CAD build for the part. Positions are in the model's coordinates, mm. Give positions to 0.01 mm unless a question says otherwise; leave off trailing zeros. Loops run counter-clockwise (first coordinate to the right, second up) from the corner with the lowest first, then second, coordinate; pieces in that order, holes last.
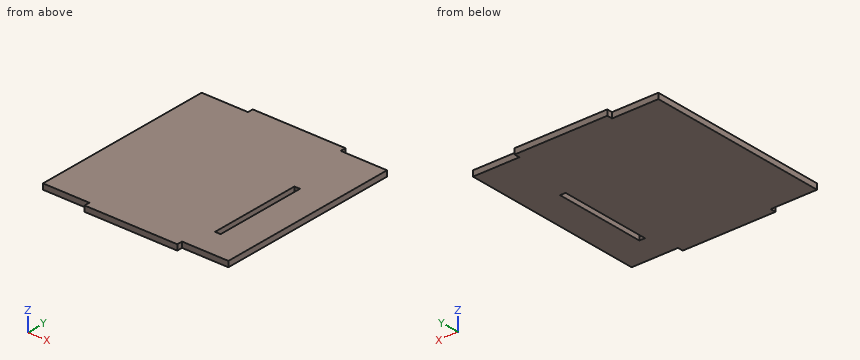
Autodesk Inventor part; units mm, degrees
ref_plane "YZ Plane" through (0, 0, 0) normal (1, 0, 0) x (0, 1, 0)
ref_plane "XZ Plane" through (0, 0, 0) normal (0, 1, 0) x (-1, 0, 0)
ref_plane "XY Plane" through (0, 0, 0) normal (0, 0, 1) x (1, 0, 0)
sketch "Boceto1" plane through (0, 0, 0) normal (0, 0, 1) x (1, 0, 0)
  line L0 (0, 100) -> (0, 0)
  line L1 (-75, 0) -> (-75, -3)
  line L2 (-75, -3) -> (-25, -3)
  line L3 (-25, -3) -> (-25, 0)
  line L4 (0, 0) -> (-25, 0)
  line L5 (-100, 0) -> (-75, 0)
  line L6 (-75, 100) -> (-75, 103)
  line L7 (-75, 103) -> (-25, 103)
  line L8 (-25, 103) -> (-25, 100)
  line L9 (0, 100) -> (-25, 100)
  line L10 (-75, 100) -> (-100, 100)
  line L11 (-100, 100) -> (-100, 0)
  dimension "d1" = 100
  dimension "d4" = 50
  dimension "d5" = 25
  dimension "d10" = 3
  dimension "d13" = 50
  dimension "d14" = 3
  dimension "d37" = 100
extrude "Extrusión2" add sketch "Boceto1" along normal blind 3
sketch "Boceto2" plane through (0, 0, 3) normal (0, 0, 1) x (1, 0, 0)
  line L0 (-20, 65) -> (-17, 65)
  line L1 (-17, 65) -> (-17, 15)
  line L2 (-17, 15) -> (-20, 15)
  line L3 (-20, 15) -> (-20, 65)
  line L4 (-25, 0) -> (0, 0)
  line L5 (-100, 100) -> (-100, 0)
  dimension "d38" = 3
  dimension "d39" = 50
  dimension "d40" = 15
  dimension "d41" = 80
extrude "Extrusión3" cut sketch "Boceto2" against normal blind 3
properties part number "Control lateral"
1. Drop flat-ended pins along their axis: pin 1 (0.9 mm diameter, centred on x = -17, z = 1.5, fed in from +Y); pin 2 (1.5 mm diameter, centred on y = 102, z = 1.5, fed in from +X). Give the stop position or say it passes through.
Responses:
pin 1: stops at y = 100
pin 2: stops at x = -25
2. Saw through at A-A, the plane y = 63. List the corners of the cut face in (x, z), and give its area (3 significant figures).
Responses:
outline: (-100, 0) - (-20, 0) - (-20, 3) - (-100, 3) - close; (-17, 0) - (0, 0) - (0, 3) - (-17, 3) - close
area: 291 mm2
3. Probe line 1 along Y through (x, z) = (-19.5, 0.7); line 2 along X through (y, z) = (37, 2.3); line 3 along Y through (x, z) = (-91, 1.75). List the from-to ranges inside material, lowest first.
Responses:
line 1: y = 0 to 15, 65 to 100
line 2: x = -100 to -20, -17 to 0
line 3: y = 0 to 100
4. Saw through at B-B, the plane z = 1.2. List the corners of the cut face in (x, y).
Responses:
outline: (-100, 0) - (-75, 0) - (-75, -3) - (-25, -3) - (-25, 0) - (0, 0) - (0, 100) - (-25, 100) - (-25, 103) - (-75, 103) - (-75, 100) - (-100, 100) - close; hole (-20, 15) - (-17, 15) - (-17, 65) - (-20, 65) - close
